Study the drawing (mm; zero at the part's minimum x, y, z) and answer. Round coordinates to 2 decimals unless told otherwise and drop trailing zeros. Write each loop counter-clockwise with the first axis right and the second up, starting at its lowest first coordinate (ties: lowest second). Pieces come first, ordered by that corner, then holes. Notation, with made-up numbers: M 31.25,9.5 L 53.25,9.5 A25 ccw 53.25,30.5 Z; hole C -13,35 d7. An arc over 180 degrees is marked long. Write each question's results on one line, items separated by ' | '.
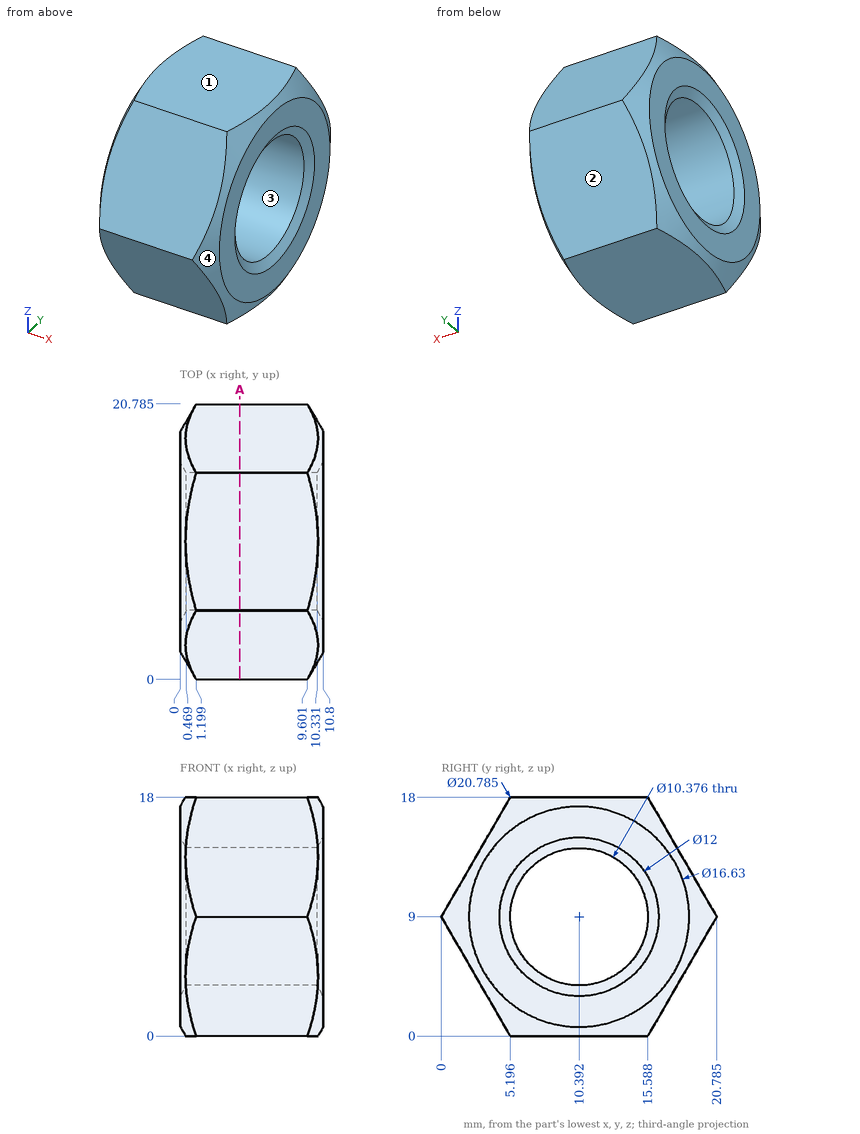
1) Find the intervals of material crossed by line 1 (Z direction, x = 2.5, y = 14); line 2 (Z direction, x = 0.75, y = 14.25) (1 decimal); line 3 (Y direction, x = 2.5, z = 8.75) (1 decimal), in increasing order.
Return value:
line 1: 0 to 5.27, 12.73 to 18 | line 2: 0.2 to 5.5, 12.5 to 17.8 | line 3: 0.1 to 5.2, 15.6 to 20.6
2) The mould has two halves that part along Y. Classify the marked faces 1, 2, 3 and 4: +Y half, -Y half, draft (parallel to the pull), parting line (faces both ways), or undercut.
Return value:
face 1: draft | face 2: +Y half | face 3: undercut | face 4: parting line
3) Section A-A (x = 4.5) is taken. Determine the outline of the cut face in (y, z) (1 decimal), then the cut area to 3 significant figures.
Return value:
outline: M 0,9 L 5.2,0 L 15.6,0 L 20.8,9 L 15.6,18 L 5.2,18 Z; hole C 10.4,9 d10.4 | area: 196 mm²
4) Each of these flat-tipped pins is pushed along its axis until it touches: pin 1 (6 mm diameter, centred on x = 9, z = 13.5, fed in from -Y) (1 decimal); pin 2 (8.5 mm diameter, centred on y = 10.39, z = 9, fed in from -X). Where does it stop, or does it pass through?
Return value:
pin 1: y = 0.9 | pin 2: through
